For this review, take the finished solid that the model builds, in its own axes (mm). A direction names the side the tool comes from. Coordinates: 2 decimals unless noted, no trailing zeros. Order: outer loops, then holes, each group sorted by start corner. A loop starts at its lowest first (then second) coordinate and runs counter-clockwise, first axis right, second up.
from build123d import *

# Parameters (mm, degrees)
CROQUIS1_W              = 4
CROQUIS1_H              = 3
CROQUIS1_W_2            = 15
CROQUIS1_H_2            = 12
SALIENTE_EXTRUIR1_DEPTH = 12
CORTAR_EXTRUIR2_DEPTH   = 12
CROQUIS5_R              = 0.81
CORTAR_EXTRUIR3_DEPTH   = 3


with BuildPart() as part:
    # Croquis1 → Saliente-Extruir1 (new body)
    with BuildSketch(Plane(origin=(0, 0, 0), x_dir=(0, 0, -1), z_dir=(1, 0, 0))):
        with Locations((-9.5, -4.5)):
            Rectangle(CROQUIS1_W, CROQUIS1_H)
        Rectangle(CROQUIS1_W_2, CROQUIS1_H_2)
        with Locations((9.5, -4.5)):
            Rectangle(CROQUIS1_W, CROQUIS1_H)
    extrude(amount=SALIENTE_EXTRUIR1_DEPTH)

    # Croquis4 → Cortar-Extruir2 (cut)
    with BuildSketch(Plane(origin=(12, 0, 0), x_dir=(0, 0, -1), z_dir=(1, 0, 0))):
        with BuildLine():
            Line((-3, -6), (3, -6))
            ThreePointArc((3, -6), (3.316227766, -5.948683298), (3.6, -5.8))
            ThreePointArc((3.6, -5.8), (6, -1), (3.6, 3.799999999))
            ThreePointArc((3.6, 3.799999999), (3.316227766, 3.948683297), (3, 3.999999999))
            Line((3, 3.999999999), (-3, 3.999999999))
            ThreePointArc((-3, 3.999999999), (-3.316227766, 3.948683297), (-3.6, 3.799999999))
            ThreePointArc((-3.6, 3.799999999), (-6, -1), (-3.6, -5.8))
            ThreePointArc((-3.6, -5.8), (-3.316227766, -5.948683298), (-3, -6))
        make_face()
    extrude(amount=-CORTAR_EXTRUIR2_DEPTH, mode=Mode.SUBTRACT)

    # Croquis5 → Cortar-Extruir3 (cut)
    with BuildSketch(Plane(origin=(0, -3, 0), x_dir=(1, 0, 0), z_dir=(0, 1, 0))):
        with Locations(Location((6, 9.5, 0), (0, 0, 270))):
            Circle(CROQUIS5_R)
        with Locations(Location((6, -9.5, 0), (0, 0, 90))):
            Circle(CROQUIS5_R)
    extrude(amount=-CORTAR_EXTRUIR3_DEPTH, mode=Mode.SUBTRACT)


solid = part.part
1. Take a section at C-C, the plane y = -5. Give the boundary of the cut face in (x, z), plus the area to 3 significant figures.
Answer below:
outline: (0, -11.5) - (12, -11.5) - (12, -4.47) - (0, -4.47) - close; (0, 4.47) - (12, 4.47) - (12, 11.5) - (0, 11.5) - close; hole circle Ø1.62 at (6, -9.5); hole circle Ø1.62 at (6, 9.5)
area: 165 mm2
2. Take a section at A-A, the plane x = 6. Give the boundary of the cut face in (y, z), plus the area to 3 significant figures.
Answer below:
outline: (-6, -11.5) - (-3, -11.5) - (-3, -10.31) - (-6, -10.31) - close; (-6, -8.69) - (-3, -8.69) - (-3, -7.5) - (6, -7.5) - (6, 7.5) - (-3, 7.5) - (-3, 8.69) - (-6, 8.69) - (-6, 3) arc R1 cw to (-5.8, 3.6) arc R6 cw to (3.8, 3.6) arc R1 cw to (4, 3) - (4, -3) arc R1 cw to (3.8, -3.6) arc R6 cw to (-5.8, -3.6) arc R1 cw to (-6, -3) - close; (-6, 10.31) - (-3, 10.31) - (-3, 11.5) - (-6, 11.5) - close
area: 90.2 mm2
3. To check wall thickness, follow L1, parallel to Z at x = 3, y = -1; L2, parallel to X at y = -4.6, z = 9.5; L3, parallel to Y at x = 11.25, z = -0.5. State the ranges of each line that lie inside material, in increasing order.
Answer below:
L1: z = -7.5 to -6, 6 to 7.5
L2: x = 0 to 5.19, 6.81 to 12
L3: y = 4 to 6
4. Machinability: for faces 1 (the face through (6, -3, -11)), 2 (the face through (6, 4, 0)), 3 (the face through (6, -1, -6)), 4 (the face through (6, -3, 8)), which of the approach directions +Z, -Z, +X, -X, +Y, -Y give a long, thin tool a straight path to every point of the face, cutting with its end or side? Answer none if there is none.
Answer below:
face 1: -Z, +X, -X, +Y
face 2: +X, -X, -Y
face 3: +X, -X
face 4: +Z, +X, -X, +Y
5. Take a section at D-D, the plane y = -1.5. Give the boundary of the cut face in (x, z), plus the area to 3 significant figures.
Answer below:
outline: (0, -7.5) - (12, -7.5) - (12, -5.98) - (0, -5.98) - close; (0, 5.98) - (12, 5.98) - (12, 7.5) - (0, 7.5) - close
area: 36.5 mm2
6. Clearance check with flat-ended pins moving along their axes: pin 1 Ø2 at (x, z) = (6, -9.5) entering from +Y; pin 2 Ø1.5 at (x, y) = (3, -1.5) entering from +Z; pin 3 Ø2 at (x, y) = (7, 1) entering from -Z. State where each tip first meets the part, or that it passes through.
Answer below:
pin 1: stops at y = -3
pin 2: stops at z = 7.5
pin 3: stops at z = -7.5
7. The part is to be moulded in two halves that separate along X. For faces 5 (the face through (5.96, -4.48, 10.31)), 6 (the face through (6, 6, 0)), 7 (the face through (12, 4.5, -0.8)), say which applies: +X half, -X half, draft (parallel to the pull), parting line (faces both ways), or undercut.
Answer below:
face 5: undercut
face 6: draft
face 7: +X half
